Part model, mm, in its own coordinate system. Give positions to 0.01 mm unless a question says otherwise; leave off trailing zeros. Order: outer loops, then holes, each group sorted by start corner. A loop starts at its lowest first (then second) coordinate and runs counter-clockwise, first axis right, second up. Notation, with made-up numbers: M 81.25,34 L 102.25,34 A14 cw 102.25,61 Z; hole C 77,24 d10. An arc over 180 degrees is marked long. Write each question's results on one line, items separated by ' | '. Start each with the question number.
Autodesk Inventor part; units mm, degrees
ref_plane "Work Plane2" through (0, -17.5, 300) normal (0, 1, 0) x (-1, 0, 0)
ref_plane "YZ Plane" through (0, 0, 0) normal (1, 0, 0) x (0, 1, 0)
ref_plane "XY Plane" through (0, 0, 0) normal (0, 0, 1) x (1, 0, 0)
sketch "Sketch1" plane through (0, 0, 0) normal (0, 1, 0) x (-1, 0, 0)
  line L0 (0, 0) -> (0, 600)
  line L1 (0, 0) -> (-17.5, 0)
  line L2 (-17.5, 0) -> (-17.5, 600)
  line L3 (-17.5, 600) -> (0, 600)
  line L4 (-17.5, 200) -> (-18, 200)
  line L5 (-18, 200) -> (-18, 350)
  line L6 (-18, 350) -> (-17.5, 350)
  dimension "d5" = 35
  dimension "d6" = 36
  dimension "d7" = 600
  dimension "d8" = 250
  dimension "d9" = 200
revolve "Revolution1" add sketch "Sketch1" angle 360 about axis through (0, 0, 0) along (0, 0, 1) contours L1 L2 L3 L0
ref_plane "Work Plane2" through (0, -17.5, 300) normal (0, 1, 0) x (-1, 0, 0)
sketch "Sketch2" plane through (0, -17.5, 300) normal (0, 1, 0) x (-1, 0, 0)
  line L0 (0, -135) -> (0, -285) construction
  line L1 (-5, -135) -> (-5, -285)
  line L2 (5, -285) -> (5, -135)
  arc A0 (5, -135) -> (-5, -135) centre (0, -135) ccw
  arc A1 (-5, -285) -> (5, -285) centre (0, -285) ccw
  point P0 (0, -300)
  point P1 (0, -210)
  point P2 (0, -290)
  dimension "d10" = 10
  dimension "d11" = 150
  dimension "d12" = 10
extrude "Extrusion1" cut sketch "Sketch2" along normal blind 5
properties part number "Вал ведущей шестерни"
(1) Drop flat-ended pins along their axis: P1, Ø10, axis at y = 7, z = 193.5, coming from the -X side; P2, Ø3.5, axis at y = -14, z = 101, coming from the +X side; P3, Ø10, axis at x = -7, z = 97, coming from the +Y side. Give the stop position or say it passes through.
(2) Saw through at A-A on x = 0. Give the cut face in (y, z), plus the area to 3 significant figures.
(3) Pull direction X, two halves, no side cores. Call faces 1 (the flat face through (0, -12.5, 91)), 2 (the flat face through (0, 0, 0)), 3 (the cylindrical face through (-2.28, 17.35, 304.2)): +X half, -X half, draft (parallel to the pull), parting line (faces both ways), or undercut.
(4) Probe L1, parallel to Y at x = 1.5, z = 207; L2, parallel to X at y = -1, z = 236.5; L3, parallel to X at y = -2, z = 128. List the from-to ranges inside material, lowest first.
(5) Saw through at B-B on z = 62.5. Give the cut face in (x, y).
(6) Saw through at C-C on y = -7.5. Give the cut face in (x, z), plus the area to 3 significant figures.
Taken from the geometry:
1) P1: stops at x = -17.39 | P2: stops at x = 12.5 | P3: stops at y = 17.39
2) outline: M -17.5,0 L 17.5,0 L 17.5,600 L -17.5,600 L -17.5,170 L -12.5,170 L -12.5,10 L -17.5,10 Z | area: 20,200 mm²
3) face 1: undercut | face 2: draft | face 3: parting line
4) L1: y = -17.44 to 17.44 | L2: x = -17.47 to 17.47 | L3: x = -17.39 to 17.39
5) outline: M -5,-16.77 L -5,-12.5 L 5,-12.5 L 5,-16.77 A17.5 ccw long Z
6) outline: M -15.81,0 L 15.81,0 L 15.81,600 L -15.81,600 Z | area: 19,000 mm²
